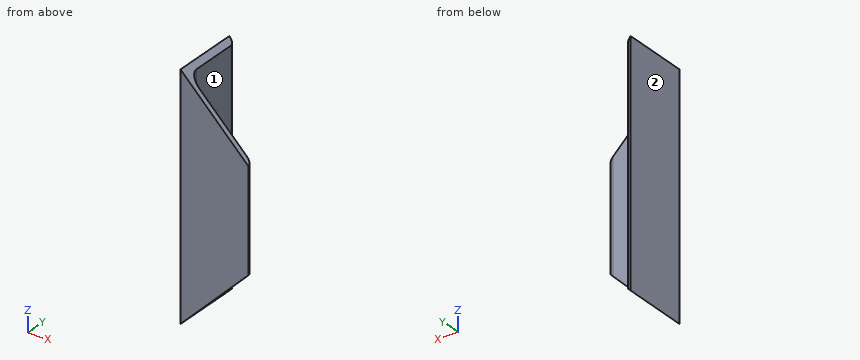
Autodesk Inventor part; units mm, degrees
ref_plane "Start plane" through (0, 0, -20) normal (0, 0, 1) x (1, 0, 0)
ref_plane "End plane" through (0, 0, 120) normal (0, 0, 1) x (1, 0, 0)
ref_plane "Work Plane11" through (-11.2, 8.8, -20) normal (0.7071, 0, -0.7071) x (-0.7071, 0, -0.7071)
ref_plane "Start plane" through (0, 0, -20) normal (0, 0, 1) x (1, 0, 0)
ref_plane "End plane" through (0, 0, 120) normal (0, 0, 1) x (1, 0, 0)
sketch "Sketch2" plane through (0, 0, 0) normal (0, 0, 1) x (1, 0, 0)
  line L0 (-8.2, -2.2) -> (-8.2, 25.8)
  line L1 (-11.2, 28.8) -> (-11.2, 28.8)
  line L2 (-11.2, -11.2) -> (-11.2, 28.8)
  line L3 (-11.2, -11.2) -> (28.8, -11.2)
  line L4 (28.8, -11.2) -> (28.8, -11.2)
  line L5 (-2.2, -8.2) -> (25.8, -8.2)
  arc A0 (-8.2, -2.2) -> (-2.2, -8.2) centre (-2.2, -2.2) ccw
  arc A1 (-8.2, 25.8) -> (-11.2, 28.8) centre (-11.2, 25.8) ccw
  arc A2 (28.8, -11.2) -> (25.8, -8.2) centre (25.8, -11.2) ccw
  line L6 (0, 37.5456) -> (0, -19.3243) construction
  line L7 (-19.3243, 0) -> (37.5456, 0) construction
  point P0 (-8.2, -8.2)
  point P1 (-8.2, 28.8)
  point P2 (28.8, -8.2)
  dimension "d4" = 40
  dimension "d6" = 40
  dimension "d8" = 3
  dimension "d10" = 3
  dimension "d17" = 6
  dimension "d18" = 3
  dimension "d19" = 11.2
  dimension "d20" = 11.2
extrude "Body" add sketch "Sketch2" along normal up to surface (140 mm away) from surface at -20
sketch "Sketch3" plane through (0, 0, 0) normal (0, 0, 1) x (1, 0, 0)
  line L0 (0, 0) -> (10, 0)
ref_plane "Work Plane10" through (0, 0, 0) normal (0, -1, 0) x (1, 0, 0)
sketch "Sketch4" plane through (0, 0, 0) normal (0, -1, 0) x (1, 0, 0)
  line L0 (-2, -20) -> (12, -20)
  line L1 (-2, 120) -> (12, 120)
  dimension "d24" = 140
ref_plane "Work Plane11" through (-11.2, 8.8, -20) normal (0.7071, 0, -0.7071) x (-0.7071, 0, -0.7071)
split "Split1" plane through (-11.2, 8.8, -20) removes the side toward (0.7071, 0, -0.7071)
ref_plane "Work Plane12" through (-11.2, 8.8, 120) normal (0.7071, 0, 0.7071) x (0.7071, 0, -0.7071)
split "Split2" plane through (-11.2, 8.8, 120) removes the side toward (0.7071, 0, 0.7071)
equation "\"d4\" = b"
equation "\"d6\" = b"
equation "\"d17\" = R"
equation "\"d18\" = R1"
equation "\"d19\" = ex"
equation "\"d20\" = d19"
equation "\"d11\" = G_L"
equation "\"b\" = 40"
equation "\"ParT\" = 3"
equation "\"R\" = 6"
equation "\"R1\" = 3"
equation "\"G_L\" = d24"
equation "\"ex\" = 11.2"
equation "\"G_OFFSET_START\" = 20"
equation "\"G_OFFSET_END\" = 20"
equation "\"d21\" = -G_OFFSET_START"
equation "\"d22\" = G_OFFSET_END + B_L"
equation "\"B_L\" = 100"
properties part number "ISO 657-1 - L40x40x3-140" material "Steel, Mild"
Design review of the part built by this model. Coordinates are the model's own, in mm. Face numbers are marked on the shaded views. A direction names the side the tool comes from. Round coordinates to 2 decimals unless told otherwise and drop trailing zeros. Write each loop counter-clockwise with the first axis right and the second up, starting at its lowest first coordinate (ties: lowest second). Pieces come first, ordered by that corner, then holes. Notation, with made-up numbers: (13.5, 55) - (49.5, 55) arc R16 cw to (49.5, 75) - close; hole circle Ø7 at (39, 17). An arc over 180 degrees is marked (long way). Return JSON: item names as keys, results as strings. Group by question number.
Item 1: We need section D-D on y = 13. Write out the cut boundary in (x, z).
Item 2: Insertion check: P1, Ø2, axis at y = 7, z = 22.5, coming from the +X side; P2, Ø6, axis at x = -4, z = 18.5, coming from the +Y side; P3, Ø8.5, axis at x = 8.5, z = 22, coming from the +Y side. Each pin has a flat end and moves straight along its axis. Give the tip position at first contact, or say it passes through.
Item 3: We need section C-C on z = 38. Write out the cut boundary in (x, y), and give its area (3 significant figures).
Item 4: Machinability: for the marked faces 1 and 2, which of the approach directions +Z, -Z, +X, -X, +Y, -Y give a long, thin tool a straight path to every point of the face, cutting with its end or side? Answer none if there is none.
Item 5: For probe 1 along Y at (x, z) = (21.5, 24.5); probe 2 along X at (y, z) = (-2.5, 66); probe 3 along Y at (x, z) = (-9, 87.5), list the stretches that pass through material, from the lowest coordinate up. Write a range as [from, to].
Item 6: We need section A-A on z = 1.5. Write out the cut boundary in (x, y).
Item 7: We need section B-B on x = 0.5. Write out the cut boundary in (y, z).
Model answer:
{
 "1": {"outline": "(-11.2, -20) - (-8.2, -17) - (-8.2, 117) - (-11.2, 120) - close"},
 "2": {"P1": "stops at x = -8.2", "P2": "stops at y = -5.8", "P3": "stops at y = -8.2"},
 "3": {"outline": "(-11.2, -11.2) - (28.8, -11.2) arc R3 ccw to (25.8, -8.2) - (-2.2, -8.2) arc R6 cw to (-8.2, -2.2) - (-8.2, 25.8) arc R3 ccw to (-11.2, 28.8) - close", "area": "235 mm²"},
 "4": {"face 1": "+Z, -Z, +X, +Y", "face 2": "+Z, -Z, -X, +Y, -Y"},
 "5": {"probe 1": "y = [-11.2, -8.2]", "probe 2": "x = [-11.2, -8.19]", "probe 3": "y = [-11.2, 27.84]"},
 "6": {"outline": "(-11.2, -11.2) - (10.3, -11.2) - (10.3, -8.2) - (-2.2, -8.2) arc R6 cw to (-8.2, -2.2) - (-8.2, 25.8) arc R3 ccw to (-11.2, 28.8) - close"},
 "7": {"outline": "(-11.2, -8.3) - (-8.2, -8.3) - (-8.2, 108.3) - (-11.2, 108.3) - close"}
}
